For this review, take the finished solid that the model builds, in its own axes (mm). Coordinates: 2 decimals unless noted, no trailing zeros. Answer as a JSON object with one key per item and string values. Group by question number.
Item 1: Wall thickness on L1, parallel to Z at x = -287, y = -2: over which ranges is the line inside the solid? List them lowest first. Write a range as from..to.
Item 2: Add section A-A (x = 0). Count the separate pieces of the cut face and the enclosed holes in it, then the cut area to 3 significant figures.
Item 3: Insertion check: pin 1 (24 mm diameter, centred on x = -174.45, z = 84.14, fed in from -Y); pin 2 (10 mm diameter, centred on x = -202, z = -53.5, fed in from +Y). Each pin has a flat end and moves straight along its axis. Give the tip position at first contact, or say it passes through.
Item 4: Mouldability with a two-part tool opening along Z and no side actions: class faces 1 (the face through (259.402, -2.028, -101.605)), 2 (the face through (170.56, -2.03, 24.8)) as +Z half, -Z half, draft (parallel to the pull), parting line (faces both ways), or undercut.
from build123d import *

# Parameters (mm, degrees)
F1_DEPTH = 4
F2_R     = 15
F3_DEPTH = 5


with BuildPart() as f1:
    # F0 (on Front) → F1 (new body)
    with BuildSketch(Plane.XZ):
        Polygon((282.5, 247.5), (0, 247.5), (-282.5, 247.5), (-282.5, 207.5), (-322.5, 207.5), (-322.5, 0), (-322.5, -207.5), (-282.5, -207.5), (-282.5, -247.5), (0, -247.5), (282.5, -247.5), (282.5, -207.5), (322.5, -207.5), (322.5, 0), (322.5, 207.5), (282.5, 207.5), align=None)
    extrude(amount=F1_DEPTH)

    # F2 (on face) → F3 (cut)
    with BuildSketch(Plane.XZ.offset(4)):
        with Locations((245.545626, -215.859562)):
            Circle(F2_R)
        with Locations((245.545626, -155.859562)):
            Circle(F2_R)
        with Locations((245.545626, -95.859562)):
            Circle(F2_R)
        with Locations((245.545626, -35.859562)):
            Circle(F2_R)
        with Locations((245.545626, 24.140438)):
            Circle(F2_R)
        with Locations((245.545626, 84.140438)):
            Circle(F2_R)
        with Locations((245.545626, 144.140438)):
            Circle(F2_R)
        with Locations((245.545626, 204.140438)):
            Circle(F2_R)
        with Locations((185.545626, -215.859562)):
            Circle(F2_R)
        with Locations((185.545626, -155.859562)):
            Circle(F2_R)
        with Locations((185.545626, -95.859562)):
            Circle(F2_R)
        with Locations((185.545626, -35.859562)):
            Circle(F2_R)
        with Locations((185.545626, 24.140438)):
            Circle(F2_R)
        with Locations((185.545626, 84.140438)):
            Circle(F2_R)
        with Locations((185.545626, 144.140438)):
            Circle(F2_R)
        with Locations((185.545626, 204.140438)):
            Circle(F2_R)
        with Locations((125.545626, -215.859562)):
            Circle(F2_R)
        with Locations((125.545626, -155.859562)):
            Circle(F2_R)
        with Locations((125.545626, -95.859562)):
            Circle(F2_R)
        with Locations((125.545626, -35.859562)):
            Circle(F2_R)
        with Locations((125.545626, 24.140438)):
            Circle(F2_R)
        with Locations((125.545626, 84.140438)):
            Circle(F2_R)
        with Locations((125.545626, 144.140438)):
            Circle(F2_R)
        with Locations((125.545626, 204.140438)):
            Circle(F2_R)
        with Locations((65.545626, -215.859562)):
            Circle(F2_R)
        with Locations((65.545626, -155.859562)):
            Circle(F2_R)
        with Locations((65.545626, -95.859562)):
            Circle(F2_R)
        with Locations((65.545626, -35.859562)):
            Circle(F2_R)
        with Locations((65.545626, 24.140438)):
            Circle(F2_R)
        with Locations((65.545626, 84.140438)):
            Circle(F2_R)
        with Locations((65.545626, 144.140438)):
            Circle(F2_R)
        with Locations((65.545626, 204.140438)):
            Circle(F2_R)
        with Locations((5.545626, -215.859562)):
            Circle(F2_R)
        with Locations((5.545626, -155.859562)):
            Circle(F2_R)
        with Locations((5.545626, -95.859562)):
            Circle(F2_R)
        with Locations((5.545626, -35.859562)):
            Circle(F2_R)
        with Locations((5.545626, 24.140438)):
            Circle(F2_R)
        with Locations((5.545626, 84.140438)):
            Circle(F2_R)
        with Locations((5.545626, 144.140438)):
            Circle(F2_R)
        with Locations((5.545626, 204.140438)):
            Circle(F2_R)
        with Locations((-54.454374, -215.859562)):
            Circle(F2_R)
        with Locations((-54.454374, -155.859562)):
            Circle(F2_R)
        with Locations((-54.454374, -95.859562)):
            Circle(F2_R)
        with Locations((-54.454374, -35.859562)):
            Circle(F2_R)
        with Locations((-54.454374, 24.140438)):
            Circle(F2_R)
        with Locations((-54.454374, 84.140438)):
            Circle(F2_R)
        with Locations((-54.454374, 144.140438)):
            Circle(F2_R)
        with Locations((-54.454374, 204.140438)):
            Circle(F2_R)
        with Locations((-114.454374, -215.859562)):
            Circle(F2_R)
        with Locations((-114.454374, -155.859562)):
            Circle(F2_R)
        with Locations((-114.454374, -95.859562)):
            Circle(F2_R)
        with Locations((-114.454374, -35.859562)):
            Circle(F2_R)
        with Locations((-114.454374, 24.140438)):
            Circle(F2_R)
        with Locations((-114.454374, 84.140438)):
            Circle(F2_R)
        with Locations((-114.454374, 144.140438)):
            Circle(F2_R)
        with Locations((-114.454374, 204.140438)):
            Circle(F2_R)
        with Locations((-174.454374, -215.859562)):
            Circle(F2_R)
        with Locations((-174.454374, -155.859562)):
            Circle(F2_R)
        with Locations((-174.454374, -95.859562)):
            Circle(F2_R)
        with Locations((-174.454374, -35.859562)):
            Circle(F2_R)
        with Locations((-174.454374, 24.140438)):
            Circle(F2_R)
        with Locations((-174.454374, 84.140438)):
            Circle(F2_R)
        with Locations((-174.454374, 144.140438)):
            Circle(F2_R)
        with Locations((-174.454374, 204.140438)):
            Circle(F2_R)
        with Locations((-234.454374, -215.859562)):
            Circle(F2_R)
        with Locations((-234.454374, -155.859562)):
            Circle(F2_R)
        with Locations((-234.454374, -95.859562)):
            Circle(F2_R)
        with Locations((-234.454374, -35.859562)):
            Circle(F2_R)
        with Locations((-234.454374, 24.140438)):
            Circle(F2_R)
        with Locations((-234.454374, 84.140438)):
            Circle(F2_R)
        with Locations((-234.454374, 144.140438)):
            Circle(F2_R)
        with Locations((-234.454374, 204.140438)):
            Circle(F2_R)
    extrude(amount=-F3_DEPTH, mode=Mode.SUBTRACT)


solid = f1.part
From the geometry:
{
 "1": {"L1": "z = -207.5..207.5"},
 "2": {"separate pieces": "9", "enclosed holes": "0", "area": "1,090 mm²"},
 "3": {"pin 1": "passes through", "pin 2": "stops at y = 0"},
 "4": {"face 1": "undercut", "face 2": "undercut"}
}
